from build123d import *

# Parameters (mm, degrees)
BOSS_EXTRUDE1_OUTLINE_W = 6.1
BOSS_EXTRUDE1_OUTLINE_H = 6.1
BOSS_EXTRUDE1_DEPTH     = 84
SKETCH1_4_R             = 2.5
BOSS_EXTRUDE2_DEPTH     = 40


# Read off the part's stored shape, not the designer's step: Boss-Extrude1
with BuildPart() as part:
    # Boss-Extrude1 outline → Boss-Extrude1 (new body)
    with BuildSketch(Plane.XY):
        Rectangle(BOSS_EXTRUDE1_OUTLINE_W, BOSS_EXTRUDE1_OUTLINE_H)
    extrude(amount=BOSS_EXTRUDE1_DEPTH)

    # Sketch1<4> → Boss-Extrude2 (add)
    with BuildSketch(Plane.XY):
        Circle(SKETCH1_4_R)
    extrude(amount=-BOSS_EXTRUDE2_DEPTH)

    # Boss-Extrude3 cone 1 section (through the dimple's axis) → Boss-Extrude3 (revolve)
    with BuildSketch(Plane(origin=(0, 0, -40), x_dir=(0, -1, 0), z_dir=(1, 0, 0))):
        Polygon((0, 0), (2.5, 0), (0, 4.330127019), align=None)
    revolve(axis=Axis((0, 0, -40), (0, 0, -1)))


solid = part.part
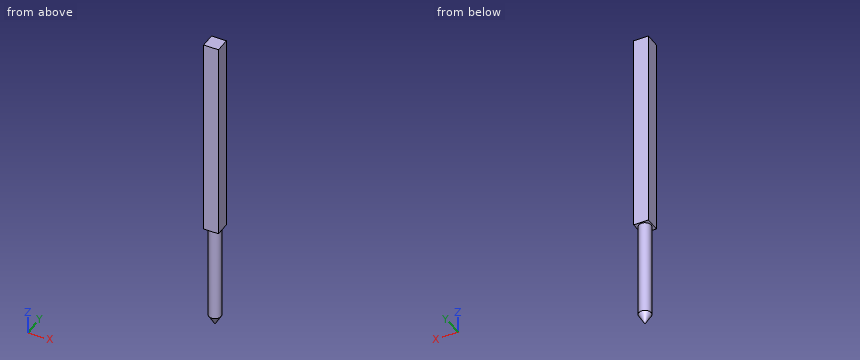
The model under review builds one solid part; all positions refer to its coordinate system, in mm. Coordinates: 2 decimals unless noted, no trailing zeros. Loops run counter-clockwise (first coordinate to the right, second up) from the corner with the lowest first, then second, coordinate; pieces in that order, holes last. Notation, with made-up numbers: M 42,46.25 L 101,46.25 A3 cw 101,51.25 Z; hole C 74.25,-10 d7. An arc over 180 degrees is marked long. Put each result on its own line as item: value. Start each with the question number.
Q1. Wall thickness on line 1 (Y direction, x = 0, z = -32); line 2 (Z direction, x = -2, y = 2.25); line 3 (X direction, y = -1.5, z = -17): over which ranges is each line inside the solid? List them lowest first.
Q2. Add section A-A (z = -34). Write out the cut boundary in (x, y).
Q3. Clearance check with flat-ended pins moving along their axes: pin 1 (3 mm diameter, centred on x = -1, y = 1.5, fed in from -Z); pin 2 (3 mm diameter, centred on x = -1.5, y = 0.5, fed in from -Z); pin 3 (1.5 mm diameter, centred on x = 1, z = -29, fed in from -Y). State where each tip first meets the part, or that it passes through.
Answers:
1. line 1: y = -2.5 to 2.5
1. line 2: z = 0 to 84
1. line 3: x = -2 to 2
2. outline: C 0,0 d5
3. pin 1: stops at z = -43.81
3. pin 2: stops at z = -44.19
3. pin 3: stops at y = -2.49
